The listing builds one solid part. Answer for the finished solid, in the listing's coordinates (mm). Coordinates: 2 decimals unless noted, no trailing zeros. Loops run counter-clockwise (first coordinate to the right, second up) from the corner with the lowest first, then second, coordinate; pieces in that order, holes last. Notation, with made-up numbers: (78.25, 44.25) - (127.25, 44.25) arc R23 ccw to (127.25, 58.25) - close; hole circle Ø7 at (53.25, 36). An arc over 180 degrees is marked (long way). Return JSON: item names as keys, results as strings. Group by question number.
1. The mould has two halves that part along Y. Classify faces 1 (the face through (-10, 6, 2)), 2 (the face through (0, -36.75, 2)), 3 (the face through (-0.26, -12.9, 1.97)): pulls with the +Y half, pulls with the -Y half, needs draft (parallel to the pull), parting line crosses it, or undercut.
2. This flat-tipped pin is pushed along its axis until it touches: P1, Ø3, axis at x = 0, y = 34.08, coming from the +Z side. Where does it stop, or does it pass through?
3. Section B-B (x = 0) is taken. State how many separate pieces and enclosed holes the cut face has, and give its area (3 significant figures).
4. Find the intervals of material crossed by line 1 along X through (y, z) = (41, 3.05); line 2 along X through (y, z) = (-12.5, 3.1), in increasing order.
5. Section A-A (y = 40.75) is taken. Write down the section's boundary in (x, z), and give its area (3 significant figures).
6. Section D-D (y = -25) is taken. Write down the section's boundary in (x, z), and give its area (3 significant figures).
Autodesk Inventor part; units mm, degrees
ref_plane "YZ Plane" through (0, 0, 0) normal (1, 0, 0) x (0, 1, 0)
ref_plane "XZ Plane" through (0, 0, 0) normal (0, 1, 0) x (-1, 0, 0)
ref_plane "XY Plane" through (0, 0, 0) normal (0, 0, 1) x (1, 0, 0)
sketch "Sketch1" plane through (0, 0, 0) normal (0, 0, 1) x (1, 0, 0)
  circle A0 centre (0, -30.375) radius 0.875
  line L0 (10, -63.625) -> (10, 47.75)
  line L1 (10, 47.75) -> (-10, 47.75)
  line L2 (-10, 47.75) -> (-10, -63.625)
  line L3 (-10, -63.625) -> (10, -63.625)
  line L4 (6.125, -36.75) -> (6.125, -59.75)
  line L5 (6.125, -59.75) -> (-6.125, -59.75)
  line L6 (-6.125, -59.75) -> (-6.125, -36.75)
  line L7 (-6.125, -36.75) -> (6.125, -36.75)
  circle A1 centre (0, 40.75) radius 2
  circle A2 centre (0, -4.25) radius 2
  circle A3 centre (0, 20.75) radius 2
  circle A4 centre (0, -24.25) radius 2
  circle A5 centre (0, 34.0833) radius 2
  circle A6 centre (0, 27.4167) radius 2
  circle A7 centre (0, -10.9167) radius 2
  circle A8 centre (0, -17.5833) radius 2
  point P0 (0, 0)
  point P1 (0, 0)
extrude "Extrusion1" add sketch "Sketch1" along normal blind 4
sketch "Sketch2" plane through (0, 0, 4) normal (0, 0, 1) x (1, 0, 0)
  line L0 (6.125, -59.75) -> (-6.125, -59.75)
  line L1 (-6.125, -59.75) -> (-6.125, -36.75)
  line L2 (-6.125, -36.75) -> (6.125, -36.75)
  line L3 (6.125, -36.75) -> (6.125, -59.75)
  circle A0 centre (0, -17.5833) radius 2
  circle A1 centre (0, -10.9167) radius 2
  circle A2 centre (0, 27.4167) radius 2
  circle A3 centre (0, 34.0833) radius 2
  circle A4 centre (0, -24.25) radius 2
  circle A5 centre (0, 20.75) radius 2
  circle A6 centre (0, -4.25) radius 2
  circle A7 centre (0, 40.75) radius 2
  circle A8 centre (0, -30.375) radius 0.875
  line L4 (10, -63.625) -> (10, 47.75)
  line L5 (10, 47.75) -> (-10, 47.75)
  line L6 (-10, 47.75) -> (-10, -63.625)
  line L7 (-10, -63.625) -> (10, -63.625)
  line L8 (-10, -36.75) -> (10, -36.75)
  point P0 (0, 0)
extrude "Extrusion2" cut sketch "Sketch2" against normal blind 4 contours L3 L8 L4 L7 L6 L1 L0
sketch "Sketch3" plane through (0, 0, 4) normal (0, 0, 1) x (1, 0, 0)
  line L0 (-10, -36.75) -> (10, -36.75)
  line L1 (10, -36.75) -> (10, 47.75)
  line L2 (10, 47.75) -> (-10, 47.75)
  line L3 (-10, 47.75) -> (-10, -36.75)
  circle A0 centre (0, -30.375) radius 0.875
  circle A1 centre (0, 40.75) radius 2
  circle A2 centre (0, -4.25) radius 2
  circle A3 centre (0, 20.75) radius 2
  circle A4 centre (0, -24.25) radius 2
  circle A5 centre (0, 34.0833) radius 2
  circle A6 centre (0, 27.4167) radius 2
  circle A7 centre (0, -10.9167) radius 2
  circle A8 centre (0, -17.5833) radius 2
  point P0 (0, 0)
extrude "Extrusion3" add sketch "Sketch3" against normal blind 4 contours A0
sketch "Sketch4" plane through (0, 0, 4) normal (0, 0, 1) x (1, 0, 0)
  line L0 (-10, -36.75) -> (10, -36.75)
  line L1 (10, -36.75) -> (10, 47.75)
  line L2 (10, 47.75) -> (-10, 47.75)
  line L3 (-10, 47.75) -> (-10, -36.75)
  circle A0 centre (0, 40.75) radius 2
  circle A1 centre (0, -4.25) radius 2
  circle A2 centre (0, 20.75) radius 2
  circle A3 centre (0, -24.25) radius 2
  circle A4 centre (0, 34.0833) radius 2
  circle A5 centre (0, 27.4167) radius 2
  circle A6 centre (0, -10.9167) radius 2
  circle A7 centre (0, -17.5833) radius 2
  line L4 (-33.7924, 18.25) -> (39.8102, 18.25) construction
  point P0 (0, 0)
  dimension "d6" = 22.5
properties part number "BottomRearLeg"
The answers:
{
 "1": {"face 1": "needs draft", "face 2": "pulls with the -Y half", "face 3": "undercut"},
 "2": {"P1": "passes through"},
 "3": {"separate pieces": "9", "enclosed holes": "0", "area": "210 mm2"},
 "4": {"line 1": "x = -10 to -1.98, 1.98 to 10", "line 2": "x = -10 to -1.22, 1.22 to 10"},
 "5": {"outline": "(-10, 0) - (-2, 0) - (-2, 4) - (-10, 4) - close; (2, 0) - (10, 0) - (10, 4) - (2, 4) - close", "area": "64.0 mm2"},
 "6": {"outline": "(-10, 0) - (-1.85, 0) - (-1.85, 4) - (-10, 4) - close; (1.85, 0) - (10, 0) - (10, 4) - (1.85, 4) - close", "area": "65.2 mm2"}
}
